Could you check a few things on this model? Use its own coordinates, in mm. Coordinates: 2 decimals unless noted, no trailing zeros. Order: outer loops, then holes, each group sorted by start corner. A loop starts at its lowest first (then second) coordinate and runs counter-clockwise, first axis right, second up. Notation, with made-up numbers: (4.5, 36.5) - (43.5, 36.5) arc R22 ccw to (43.5, 52.5) - close; hole circle Ø6 at (34.25, -33). An arc over 180 degrees is marked (long way). One line per item, written item: value. Start each with the question number.
from build123d import *

# Parameters (mm, degrees)
SKETCH1_R                 = 93.6625
SKETCH1_R_2               = 87.3125
BOSS_EXTRUDE1_DEPTH       = 6.35
BOSS_EXTRUDE2_DEPTH       = 6.35
SKETCH4_W                 = 173.355
SKETCH4_H                 = 4.7625
SKETCH4_W_2               = 177.8
CUT_EXTRUDE2_DEPTH        = 6.35
F_6_CLEARANCE_HOLE1_D     = 3.7973
F_6_CLEARANCE_HOLE1_DEPTH = 25.4
F_6_CLEARANCE_HOLE1_TIP   = 1.140824014


with BuildPart() as part:
    # Sketch1 → Boss-Extrude1 (new body)
    with BuildSketch(Plane.XY):
        Circle(SKETCH1_R)
        Circle(SKETCH1_R_2, mode=Mode.SUBTRACT)
    extrude(amount=BOSS_EXTRUDE1_DEPTH)

    # Sketch3 → Boss-Extrude2 (add, through all)
    with BuildSketch(Plane.XY.offset(6.35)):
        with BuildLine():
            ThreePointArc((-66.063141847, 57.08882505), (-57.249132772, 57.249132772), (-57.08882505, 66.063141847))
            ThreePointArc((-57.08882505, 66.063141847), (-61.739260832, 61.739260832), (-66.063141847, 57.08882505))
        make_face()
        with BuildLine():
            ThreePointArc((6.345800264, 87.081590909), (0, 87.3125), (-6.345800264, 87.081590909))
            ThreePointArc((-6.345800264, 87.081590909), (0, 80.9625), (6.345800264, 87.081590909))
        make_face()
        with BuildLine():
            ThreePointArc((66.063141847, 57.08882505), (61.739260832, 61.739260832), (57.08882505, 66.063141847))
            ThreePointArc((57.08882505, 66.063141847), (57.249132772, 57.249132772), (66.063141847, 57.08882505))
        make_face()
        with BuildLine():
            ThreePointArc((87.3125, 0), (87.254753631, 3.175), (87.081590909, 6.345800264))
            ThreePointArc((87.081590909, 6.345800264), (80.9625, 0), (87.081590909, -6.345800264))
            ThreePointArc((87.081590909, -6.345800264), (87.254753631, -3.175), (87.3125, 0))
        make_face()
        with BuildLine():
            ThreePointArc((57.08882505, -66.063141847), (61.739260832, -61.739260832), (66.063141847, -57.08882505))
            ThreePointArc((66.063141847, -57.08882505), (57.249132772, -57.249132772), (57.08882505, -66.063141847))
        make_face()
        with BuildLine():
            ThreePointArc((6.345800264, -87.081590909), (0, -80.9625), (-6.345800264, -87.081590909))
            ThreePointArc((-6.345800264, -87.081590909), (0, -87.3125), (6.345800264, -87.081590909))
        make_face()
        with BuildLine():
            ThreePointArc((-57.08882505, -66.063141847), (-57.249132772, -57.249132772), (-66.063141847, -57.08882505))
            ThreePointArc((-66.063141847, -57.08882505), (-61.739260832, -61.739260832), (-57.08882505, -66.063141847))
        make_face()
        with BuildLine():
            ThreePointArc((-87.081590909, -6.345800264), (-80.9625, 0), (-87.081590909, 6.345800264))
            ThreePointArc((-87.081590909, 6.345800264), (-87.3125, 0), (-87.081590909, -6.345800264))
        make_face()
    extrude(amount=-BOSS_EXTRUDE2_DEPTH)

    # Sketch4 → Cut-Extrude2 (cut)
    with BuildSketch(Plane.XY.offset(6.35)):
        with Locations((0, 30.95625)):
            Rectangle(SKETCH4_W, SKETCH4_H)
        Rectangle(SKETCH4_W_2, SKETCH4_H)
        with Locations((0, -30.95625)):
            Rectangle(SKETCH4_W, SKETCH4_H)
    extrude(amount=-CUT_EXTRUDE2_DEPTH, mode=Mode.SUBTRACT)

    # #6 Clearance Hole1
    with Locations(Plane.XY.offset(6.35)):
        with Locations((-87.081590909, 0), (-61.575983448, 61.575983448), (0, 87.081590909), (61.575983448, 61.575983448), (87.081590909, 0), (61.575983448, -61.575983448), (0, -87.081590909), (-61.575983448, -61.575983448)):
            Hole(F_6_CLEARANCE_HOLE1_D / 2, depth=F_6_CLEARANCE_HOLE1_DEPTH)
            with Locations((0, 0, -(F_6_CLEARANCE_HOLE1_DEPTH + F_6_CLEARANCE_HOLE1_TIP / 2))):  # 118° drill point
                Cone(0, F_6_CLEARANCE_HOLE1_D / 2, F_6_CLEARANCE_HOLE1_TIP, mode=Mode.SUBTRACT)


solid = part.part
Q1. We'd pull the mould along X, two halves only. Please class faces 1 (the cylindrical face through (-85.55, -17.45, 3.13)), 2 (the flat face through (-56, 63, 6.35)): +X half, -X half, draft (parallel to the pull), parting line (faces both ways), or undercut.
Q2. I want a section at B-B on x = -16.5. Please give me the cut outline in (y, z), then the cut area to 3 significant figures.
Q3. I'm going to push flat-ended pins straight in: pin 1 (1.4 mm diameter, centred on y = -32, z = 3.5, fed in from -X); pin 2 (1.4 mm diameter, centred on y = -30.5, z = 3, fed in from +X); pin 3 (2 mm diameter, centred on x = 85.5, z = 3.5, fed in from +Y); pin 4 (6 mm diameter, centred on x = -61.58, y = 61.58, fed in from -Z). Where does each tip first touch, or does it pass through?
Q4. I want a section at C-C on z = 2. State how many separate pieces and enclosed holes the cut face has, then the cut area to 3 significant figures.
Q5. I want a section at A-A on y = -76.5. Please give me the cut outline in (x, z), then the cut area to 3 significant figures.
Q6. If I drill on L1, parallel to Y at x = 0, z = 4.25; L2, parallel to Y at x = 61, z = 4; L3, parallel to X at y = 2.5, z = 4.5, over which ranges is the centre line in solid material (lowest first)?
Values follow:
1. face 1: undercut
1. face 2: draft
2. outline: (-92.2, 0) - (-85.74, 0) - (-85.74, 6.35) - (-92.2, 6.35) - close; (85.74, 0) - (92.2, 0) - (92.2, 6.35) - (85.74, 6.35) - close
2. area: 82.0 mm^2
3. pin 1: stops at x = -88.28
3. pin 2: stops at x = 88.8
3. pin 3: stops at y = 40.4
3. pin 4: stops at z = 0
4. separate pieces: 1
4. enclosed holes: 7
4. area: 3,870 mm^2
5. outline: (-54.04, 0) - (-42.09, 0) - (-42.09, 6.35) - (-54.04, 6.35) - close; (42.09, 0) - (54.04, 0) - (54.04, 6.35) - (42.09, 6.35) - close
5. area: 152 mm^2
6. L1: y = -93.66 to -88.98, -85.18 to -80.96, 80.96 to 85.18, 88.98 to 93.66
6. L2: y = -71.08 to -63.39, -59.77 to -55.43, 55.43 to 59.77, 63.39 to 71.08
6. L3: x = -93.63 to -81.48, 81.48 to 93.63
